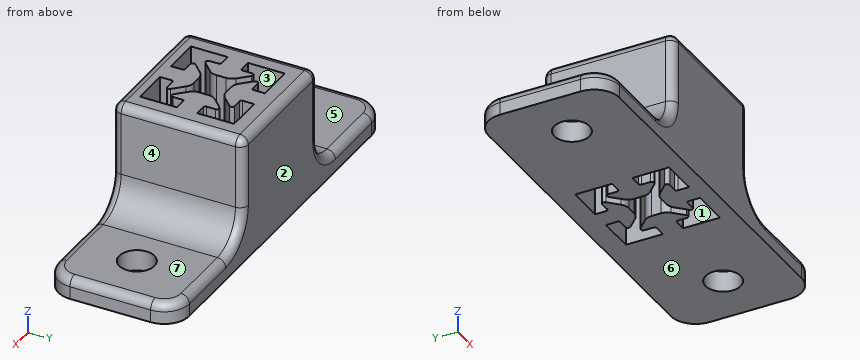
```python
from build123d import *

# Parameters (mm, degrees)
SKETCH2_W           = 32.4
SKETCH2_H           = 31.2
BOSS_EXTRUDE1_DEPTH = 30
SKETCH3_W           = 5
SKETCH3_H           = 31.2
BOSS_EXTRUDE2_DEPTH = 30
SKETCH4_R           = 4.198469776
CUT_EXTRUDE1_DEPTH  = 15
FILLET6_R           = 8
FILLET7_R           = 6
FILLET8_R           = 2


with BuildPart() as part:
    # Sketch2 → Boss-Extrude1 (new body)
    with BuildSketch(Plane.XY.offset(-585.734831934)):
        with Locations((-220.618842126, 630.6)):
            Rectangle(SKETCH2_W, SKETCH2_H)
        with BuildLine():
            Line((-218.223842126, 639.2), (-218.223842126, 638.500000763))
            ThreePointArc((-218.223842126, 638.500000763), (-218.083253443, 638.160589569), (-217.743842299, 638.020000763))
            Line((-217.743842299, 638.020000763), (-215.574720714, 638.019999981))
            ThreePointArc((-215.574720714, 638.019999981), (-215.020393169, 637.649609941), (-215.150456861, 636.995735913))
            Line((-215.150456861, 636.995735913), (-217.490233892, 634.655958882))
            ThreePointArc((-217.490233892, 634.655958882), (-218.405107733, 634.044659724), (-219.484275009, 633.830000005))
            Line((-219.484275009, 633.830000005), (-221.753409227, 633.83))
            ThreePointArc((-221.753409227, 633.83), (-222.83257651, 634.044659717), (-223.747450356, 634.655958877))
            Line((-223.747450356, 634.655958877), (-226.087227386, 636.995735907))
            ThreePointArc((-226.087227386, 636.995735907), (-226.217291078, 637.649609934), (-225.662963535, 638.019999975))
            Line((-225.662963535, 638.019999975), (-223.493841952, 638.020000763))
            ThreePointArc((-223.493841952, 638.020000763), (-223.15443081, 638.16058957), (-223.013842126, 638.500000763))
            Line((-223.013842126, 638.500000763), (-223.013842126, 639.2))
            Line((-223.013842126, 639.2), (-223.013842126, 641.2))
            Line((-223.013842126, 641.2), (-231.818842126, 641.2))
            Line((-231.818842126, 641.2), (-231.818842126, 632.395))
            Line((-231.818842126, 632.395), (-229.818842126, 632.395))
            Line((-229.818842126, 632.395), (-229.118842889, 632.395))
            ThreePointArc((-229.118842889, 632.395), (-228.779431696, 632.535588684), (-228.638842889, 632.874999827))
            Line((-228.638842889, 632.874999827), (-228.638842108, 635.044121413))
            ThreePointArc((-228.638842108, 635.044121413), (-228.268452067, 635.598448957), (-227.614578039, 635.468385265))
            Line((-227.614578039, 635.468385265), (-225.274801008, 633.128608235))
            ThreePointArc((-225.274801008, 633.128608235), (-224.663501851, 632.213734394), (-224.448842131, 631.134567117))
            Line((-224.448842131, 631.134567117), (-224.448842127, 628.865432899))
            ThreePointArc((-224.448842127, 628.865432899), (-224.663501844, 627.786265617), (-225.274801004, 626.87139177))
            Line((-225.274801004, 626.87139177), (-227.614578033, 624.531614741))
            ThreePointArc((-227.614578033, 624.531614741), (-228.268452061, 624.401551048), (-228.638842102, 624.955878592))
            Line((-228.638842102, 624.955878592), (-228.638842889, 627.125000174))
            ThreePointArc((-228.638842889, 627.125000174), (-228.779431696, 627.464411317), (-229.118842889, 627.605))
            Line((-229.118842889, 627.605), (-229.818842126, 627.605))
            Line((-229.818842126, 627.605), (-231.818842126, 627.605))
            Line((-231.818842126, 627.605), (-231.818842126, 618.8))
            Line((-231.818842126, 618.8), (-223.013842126, 618.8))
            Line((-223.013842126, 618.8), (-223.013842126, 620.8))
            Line((-223.013842126, 620.8), (-223.013842126, 621.499999237))
            ThreePointArc((-223.013842126, 621.499999237), (-223.15443081, 621.839410431), (-223.493841954, 621.979999237))
            Line((-223.493841954, 621.979999237), (-225.662963539, 621.980000019))
            ThreePointArc((-225.662963539, 621.980000019), (-226.217291084, 622.350390059), (-226.087227392, 623.004264087))
            Line((-226.087227392, 623.004264087), (-223.747450361, 625.344041118))
            ThreePointArc((-223.747450361, 625.344041118), (-222.83257652, 625.955340276), (-221.753409244, 626.169999995))
            Line((-221.753409244, 626.169999995), (-219.484275025, 626.17))
            ThreePointArc((-219.484275025, 626.17), (-218.405107743, 625.955340283), (-217.490233897, 625.344041123))
            Line((-217.490233897, 625.344041123), (-215.150456867, 623.004264093))
            ThreePointArc((-215.150456867, 623.004264093), (-215.020393175, 622.350390066), (-215.574720718, 621.980000025))
            Line((-215.574720718, 621.980000025), (-217.743842301, 621.979999237))
            ThreePointArc((-217.743842301, 621.979999237), (-218.083253443, 621.83941043), (-218.223842126, 621.499999237))
            Line((-218.223842126, 621.499999237), (-218.223842126, 620.8))
            Line((-218.223842126, 620.8), (-218.223842126, 618.8))
            Line((-218.223842126, 618.8), (-209.418842126, 618.8))
            Line((-209.418842126, 618.8), (-209.418842126, 627.605))
            Line((-209.418842126, 627.605), (-211.418842126, 627.605))
            Line((-211.418842126, 627.605), (-212.118841364, 627.605))
            ThreePointArc((-212.118841364, 627.605), (-212.458252557, 627.464411316), (-212.598841364, 627.125000173))
            Line((-212.598841364, 627.125000173), (-212.598842145, 624.955878587))
            ThreePointArc((-212.598842145, 624.955878587), (-212.969232185, 624.401551043), (-213.623106214, 624.531614735))
            Line((-213.623106214, 624.531614735), (-215.962883245, 626.871391765))
            ThreePointArc((-215.962883245, 626.871391765), (-216.574182402, 627.786265606), (-216.788842122, 628.865432883))
            Line((-216.788842122, 628.865432883), (-216.788842126, 631.134567101))
            ThreePointArc((-216.788842126, 631.134567101), (-216.574182409, 632.213734383), (-215.962883249, 633.12860823))
            Line((-215.962883249, 633.12860823), (-213.62310622, 635.468385259))
            ThreePointArc((-213.62310622, 635.468385259), (-212.969232192, 635.598448952), (-212.598842151, 635.044121408))
            Line((-212.598842151, 635.044121408), (-212.598841364, 632.874999826))
            ThreePointArc((-212.598841364, 632.874999826), (-212.458252557, 632.535588683), (-212.118841364, 632.395))
            Line((-212.118841364, 632.395), (-211.418842126, 632.395))
            Line((-211.418842126, 632.395), (-209.418842126, 632.395))
            Line((-209.418842126, 632.395), (-209.418842126, 641.2))
            Line((-209.418842126, 641.2), (-218.223842126, 641.2))
            Line((-218.223842126, 641.2), (-218.223842126, 639.2))
        make_face(mode=Mode.SUBTRACT)
    extrude(amount=BOSS_EXTRUDE1_DEPTH)

    # Sketch3 → Boss-Extrude2 (add)
    with BuildSketch(Plane(origin=(-204.418842126, 0, 0), x_dir=(0, 0, -1), z_dir=(1, 0, 0))):
        with Locations((583.234831934, 630.6)):
            Rectangle(SKETCH3_W, SKETCH3_H)
    boss_extrude2 = extrude(amount=BOSS_EXTRUDE2_DEPTH)

    # Sketch4 → Cut-Extrude1 (cut, symmetric)
    with BuildSketch(Plane.XY.offset(-580.734831934)):
        with Locations((-187.243842126, 630)):
            Circle(SKETCH4_R)
    cut_extrude1 = extrude(amount=CUT_EXTRUDE1_DEPTH, both=True, mode=Mode.SUBTRACT)

    # Mirror6: Boss-Extrude2 across plane
    add(boss_extrude2.mirror(Plane(origin=(-220.618842126, 0, 0), x_dir=(0, 0, 1), z_dir=(1, 0, 0))))

    # Mirror9: Cut-Extrude1 across plane
    add(cut_extrude1.mirror(Plane(origin=(-220.618842126, 0, 0), x_dir=(0, 0, 1), z_dir=(1, 0, 0))), mode=Mode.SUBTRACT)

    # Fillet6
    fillet6_edges = [part.edges().sort_by_distance(p)[0] for p in [
        (-204.418842126, 630.6, -580.734831934),
        (-236.818842126, 630.6, -580.734831934),
    ]]
    fillet(fillet6_edges, radius=FILLET6_R)

    # Fillet7
    fillet7_edges = [part.edges().sort_by_distance(p)[0] for p in [
        (-174.418842126, 646.2, -583.234831934),
        (-174.418842126, 615, -583.234831934),
        (-266.818842126, 615, -583.234831934),
        (-266.818842126, 646.2, -583.234831934),
    ]]
    fillet(fillet7_edges, radius=FILLET7_R)

    # Fillet8
    fillet8_edges = [part.edges().sort_by_distance(p)[0] for p in [
        (-204.418842126, 630.6, -555.734831934),
        (-220.618842126, 646.2, -555.734831934),
        (-239.161987877, 615, -578.391686183),
        (-239.161987877, 646.2, -578.391686183),
        (-202.075696376, 615, -578.391686183),
        (-202.075696376, 646.2, -578.391686183),
        (-188.418842126, 615, -580.734831934),
        (-252.818842126, 615, -580.734831934),
        (-266.818842126, 630.6, -580.734831934),
        (-252.818842126, 646.2, -580.734831934),
        (-265.061482814, 644.442640687, -580.734831934),
        (-265.061482814, 616.757359313, -580.734831934),
        (-188.418842126, 646.2, -580.734831934),
        (-174.418842126, 630.6, -580.734831934),
        (-176.176201439, 644.442640687, -580.734831934),
        (-176.176201439, 616.757359313, -580.734831934),
        (-236.818842126, 630.6, -555.734831934),
        (-236.818842126, 646.2, -564.234831934),
        (-204.418842126, 646.2, -564.234831934),
        (-204.418842126, 615, -564.234831934),
        (-236.818842126, 615, -564.234831934),
        (-220.618842126, 615, -555.734831934),
    ]]
    fillet(fillet8_edges, radius=FILLET8_R)


solid = part.part
```
CAD build for the part. Positions are in the model's coordinates, mm. Face numbers are marked on the shaded views. A direction names the side the tool comes from. Round coordinates to 2 decimals unless told otherwise and drop trailing zeros. Write each loop counter-clockwise with the first axis right and the second up, starting at its lowest first coordinate (ties: lowest second). Pieces come first, ordered by that corner, then holes. Notation, with made-up numbers: (77, -32) - (87, -32) arc R29 ccw to (87, -9) - close; hole circle Ø5 at (74, 11). An arc over 180 degrees is marked (long way). Return JSON: item names as keys, results as strings. Group by question number.
Item 1: Mould opens along Y. For the marked faces 1, 2, 3 and 4 say: +Y half, -Y half, draft (parallel to the pull), parting line (faces both ways), or undercut.
Item 2: Band-saw the part on B-B on x = -184. List the corners of the cut face in (y, z), plus the area to 3 significant figures.
Item 3: Probe probe 1 along X at (y, z) = (630, -584.15); probe 2 along X at (y, z) = (640.5, -573); probe 3 along Y at (x, z) = (-231, -559.25) (3 decimals). List the from-to ranges inside material, lowest first.
Item 4: 3-axis set-ups, long thin cutter, end or side, ignore diameter. For the marked faces 5, 6 and 7: which of +Z, -Z, +X, -X, +Y, -Y reach the whole face in a straight line?
Item 5: Band-saw the part on A-A on y = 630. List the corners of the cut face in (x, z).
Item 6: Flat gauge pins, fed straight in: pin 1 Ø10 at (x, y) = (-224.5, 634) entering from +Z; pin 2 Ø2.5 at (y, z) = (626.5, -574.5) entering from -X; pin 3 Ø0.7 at (y, z) = (634, -563) entering from -X; pin 4 Ø0.8 at (y, z) = (639.5, -567.5) entering from +X. Where does each tip first touch, or does it go through?
Resolved:
{
 "1": {"face 1": "undercut", "face 2": "+Y half", "face 3": "undercut", "face 4": "draft"},
 "2": {"outline": "(615, -585.73) - (627.33, -585.73) - (627.33, -580.73) - (617, -580.73) arc R2 ccw to (615, -582.73) - close; (632.67, -585.73) - (646.2, -585.73) - (646.2, -582.73) arc R2 ccw to (644.2, -580.73) - (632.67, -580.73) - close", "area": "128 mm²"},
 "3": {"probe 1": "x = -266.82 to -258.19, -249.8 to -224.45, -216.79 to -191.44, -183.05 to -174.42", "probe 2": "x = -236.82 to -231.82, -223.01 to -218.22, -209.42 to -204.41", "probe 3": "y = 615 to 618.8, 627.605 to 632.395, 641.2 to 646.2"},
 "4": {"face 5": "+Z, -X, +Y, -Y", "face 6": "-Z, +X, -X, +Y, -Y", "face 7": "+Z, +X, +Y, -Y"},
 "5": {"outline": "(-266.82, -585.73) - (-258.19, -585.73) - (-258.19, -580.73) - (-264.82, -580.73) arc R2 ccw to (-266.82, -582.73) - close; (-249.8, -585.73) - (-224.45, -585.73) - (-224.45, -555.73) - (-234.82, -555.73) arc R2 ccw to (-236.82, -557.73) - (-236.82, -572.73) arc R8 cw to (-244.82, -580.73) - (-249.8, -580.73) - close; (-216.79, -585.73) - (-191.44, -585.73) - (-191.44, -580.73) - (-196.42, -580.73) arc R8 cw to (-204.42, -572.73) - (-204.42, -557.73) arc R2 ccw to (-206.42, -555.73) - (-216.79, -555.73) - close; (-183.05, -585.73) - (-174.42, -585.73) - (-174.42, -582.73) arc R2 ccw to (-176.42, -580.73) - (-183.05, -580.73) - close"},
 "6": {"pin 1": "stops at z = -555.73", "pin 2": "stops at x = -237.41", "pin 3": "stops at x = -236.82", "pin 4": "stops at x = -204.42"}
}
